Here's how the part is built. I have some questions about the finished solid (model axes, mm). A direction names the side the tool comes from. Coordinates: 2 decimals unless noted, no trailing zeros. Loops run counter-clockwise (first coordinate to the right, second up) from the corner with the lowest first, then second, coordinate; pieces in that order, holes last. Notation, with made-up numbers: M 71.25,71.25 L 120.25,71.25 A26 ccw 120.25,94.25 Z; hole C 18,29.25 d3. An arc over 180 degrees is marked long. Use one line per item in the form item = value. Start each with the question number.
(1) Will these pins go through, and if not, where does the flat tip stop? P1, Ø1.3, axis at x = 0, z = 7, coming from the +Y side; P2, Ø1.5, axis at y = 1.5, z = 4, coming from the -X side.
(2) Imagine slicing it at C-C, the plane z = 7.25. Please give me the cut outline in (x, y), and give its area (3 significant figures).
(3) Please list where these lines run through material, in increasing order: L1, parallel to X at y = 2.85, z = 0 (3 decimals); L2, parallel to X at y = 2.9, z = 4.25; L3, parallel to X at y = 3.35, z = -5.25.
(4) Imagine slicing it at A-A, the plane x = 0. Please give me the cut outline in (y, z) (3 decimals), and give its area (3 significant figures).
(5) Thinking about a two-plate mould opening in Z: for faces 3 (the cylindrical face through (2.703, 2.071, 8.584)), 4 (the cylindrical face through (-3.834, 2.129, -5.096)), 5 (the flat face through (-4, 0, 0)), which applies, +Z half, -Z half, draft (parallel to the pull), parting line (faces both ways), or undercut?
(6) On a 3-axis mill with a long thin cutter (end or side, diameter ignored), from which of +Z, -Z, +X, -X, +Y, -Y can I reach the whole of each face in a straight line? I mean faces 1 (the cylindrical face through (0.9, 1.82, -2.86)), 2 (the cylindrical face through (-6.662, 2.129, 1.073)). Say none if no direction works.
(7) Imagine slicing it at B-B, the plane z = 0. Please give me the cut outline in (x, y) (3 decimals).
(8) Imagine slicing it at D-D, the plane y = 1.45. State how many separate pieces and enclosed holes the cut face has, and give its area (3 significant figures).
```python
from build123d import *

# Parameters (mm, degrees)
SKETCH1_R                = 9
BRACKETMOUNT_DEPTH       = 4.2
SKETCH2_R                = 1.125
BRACKET_MOUNTHOLES_DEPTH = 4.2
SKETCH3_R                = 3
AXLEHOLE_DEPTH           = 3.7


with BuildPart() as part:
    # Sketch1 → BracketMount (new body)
    with BuildSketch(Plane(origin=(0, 0, 0), x_dir=(1, 0, 0), z_dir=(0, 1, 0))):
        with Locations(Location((0, 0, 0), (0, 0, 270))):
            Circle(SKETCH1_R)
    extrude(amount=BRACKETMOUNT_DEPTH)

    # Sketch2 → Bracket-MountHoles (cut)
    with BuildSketch(Plane(origin=(0, 4.2, 0), x_dir=(1, 0, 0), z_dir=(0, 1, 0))):
        with Locations(Location((0, 7, 0), (0, 0, 270))):
            Circle(SKETCH2_R)
        with Locations(Location((4.949747468, 4.949747468, 0), (0, 0, 270))):
            Circle(SKETCH2_R)
        with Locations(Location((7, 0, 0), (0, 0, 270))):
            Circle(SKETCH2_R)
        with Locations(Location((4.949747468, -4.949747468, 0), (0, 0, 270))):
            Circle(SKETCH2_R)
        with Locations(Location((0, -7, 0), (0, 0, 270))):
            Circle(SKETCH2_R)
        with Locations(Location((-4.949747468, -4.949747468, 0), (0, 0, 270))):
            Circle(SKETCH2_R)
        with Locations(Location((-7, 0, 0), (0, 0, 270))):
            Circle(SKETCH2_R)
        with Locations(Location((-4.949747468, 4.949747468, 0), (0, 0, 270))):
            Circle(SKETCH2_R)
    extrude(amount=-BRACKET_MOUNTHOLES_DEPTH, mode=Mode.SUBTRACT)

    # Sketch3 → AxleHole (cut)
    with BuildSketch(Plane.XZ):
        with Locations(Location((0, 0, 0), (0, 0, 270))):
            Circle(SKETCH3_R)
    extrude(amount=-AXLEHOLE_DEPTH, mode=Mode.SUBTRACT)


solid = part.part
```
Answer:
q1.P1 = through
q1.P2 = -8.39
q2.outline = M -5.33,0 L -1.1,0 L -1.1,4.2 L -5.33,4.2 Z; M 1.1,0 L 5.33,0 L 5.33,4.2 L 1.1,4.2 Z
q2.area = 35.6 mm²
q3.L1 = -9 to -8.125, -5.875 to -3, 3 to 5.875, 8.125 to 9
q3.L2 = -7.93 to -5.83, -4.07 to 4.07, 5.83 to 7.93
q3.L3 = -7.31 to -6.03, -3.87 to 3.87, 6.03 to 7.31
q4.outline = M 0,-9 L 4.2,-9 L 4.2,-8.125 L 0,-8.125 Z; M 0,-5.875 L 4.2,-5.875 L 4.2,5.875 L 0,5.875 L 0,3 L 3.7,3 L 3.7,-3 L 0,-3 Z; M 0,8.125 L 4.2,8.125 L 4.2,9 L 0,9 Z
q4.area = 34.5 mm²
q5.face_3 = parting line
q5.face_4 = undercut
q5.face_5 = draft
q6.face_1 = -Y
q6.face_2 = +Y, -Y
q7.outline = M -9,0 L -8.125,0 L -8.125,4.2 L -9,4.2 Z; M -5.875,0 L -3,0 L -3,3.7 L 3,3.7 L 3,0 L 5.875,0 L 5.875,4.2 L -5.875,4.2 Z; M 8.125,0 L 9,0 L 9,4.2 L 8.125,4.2 Z
q8.separate_pieces = 1
q8.enclosed_holes = 9
q8.area = 194 mm²
